```python
from build123d import *

# Parameters (mm, degrees)
F0_W     = 15
F0_H     = 15
F1_DEPTH = 15
F2_SIZE  = 13
F3_R     = 5.25
F3_R_2   = 2.25
F4_DEPTH = 5
F5_DEPTH = 3


with BuildPart() as f1:
    # F0 (on Top) → F1 (new body)
    with BuildSketch(Plane.XY):
        with Locations((7.5, -7.5)):
            Rectangle(F0_W, F0_H)
    extrude(amount=F1_DEPTH)

    # F2
    f2_edges = [f1.edges().sort_by_distance(p)[0] for p in [
        (15, -7.5, 15),
    ]]
    chamfer(f2_edges, length=F2_SIZE)

    # F3 (on face) → F4 (cut)
    with BuildSketch(Plane(origin=(8.5, 0, 8.5), x_dir=(0, 1, 0), z_dir=(0.7071067812, 0, 0.7071067812))):
        with Locations((-7.5, 0)):
            Circle(F3_R)
        with Locations((-7.5, 0)):
            Circle(F3_R_2, mode=Mode.SUBTRACT)
    extrude(amount=-F4_DEPTH, mode=Mode.SUBTRACT)

    # F5 (cut): a face of the model
    f5_faces = [f1.faces().sort_by_distance(p)[0] for p in [
        (8.5, -7.5, 8.5),
    ]]
    extrude(f5_faces, amount=-F5_DEPTH, mode=Mode.SUBTRACT)


solid = f1.part
```
Work out the finished part from the listing and answer in its coordinate system (mm). A direction names the side the tool comes from. Give positions to 0.01 mm unless a question says otherwise; leave off trailing zeros. Write each loop counter-clockwise with the first axis right and the second up, starting at its lowest first coordinate (ties: lowest second). Pieces come first, ordered by that corner, then holes. Notation, with made-up numbers: (1, -13.75) - (20, -13.75) arc R19 ccw to (20, -7.75) - close; hole circle Ø4 at (0.5, 82.25). An arc over 180 degrees is marked (long way). Use one line per item in the form item = value.
1. Consider L1, parallel to Z at x = 3, y = -3.25; L2, parallel to Z at x = 2.25, y = -5.25; L3, parallel to Y at x = 4, z = 8. Determine where each line is inside the solid, lowest interval first.
Filled in:
L1 = 0 to 6.93, 7.36 to 14
L2 = 0 to 7.68, 8.96 to 14.75
L3 = -15 to -11.92, -3.08 to 0
2. A cutting plane is placed at A-A (y = -8.25). Write down the section's boundary in (x, z).
Filled in:
outline = (0, 0) - (15, 0) - (15, 2) - (12.17, 4.83) - (8.64, 1.29) - (6.46, 3.46) - (7.88, 4.88) - (4.88, 7.88) - (3.46, 6.46) - (1.29, 8.64) - (4.83, 12.17) - (2, 15) - (0, 15) - close
3. A cutting plane is placed at B-B (x = 13). Write down the section's boundary in (y, z).
Filled in:
outline = (-15, 0) - (0, 0) - (0, 4) - (-15, 4) - close
4. For faces 5 (the face through (6.36, -7.53, 6.4)), 6 (the face through (1, -7, 15)), determine the directions among +Z, -Z, +X, -X, +Y, -Y from which every point of the face is accessible in a straight line to the end or side of a thin tool.
Filled in:
face_5 = +Z, +X
face_6 = +Z, +X, -X, +Y, -Y
5. A cutting plane is placed at C-C (z = 12.5). Write down the section's boundary in (x, y), and give its area (3 significant figures).
Filled in:
outline = (0, -15) - (4.5, -15) - (4.5, 0) - (0, 0) - close
area = 67.5 mm^2
6. A cutting plane is placed at D-D (y = -2.5). Write down the section's boundary in (x, z).
Filled in:
outline = (0, 0) - (15, 0) - (15, 2) - (9.63, 7.37) - (6.1, 3.83) - (3.83, 6.1) - (7.37, 9.63) - (2, 15) - (0, 15) - close
7. Each of these flat-tipped pins is pushed along its axis until it touches: pin 1 Ø5 at (y, z) = (-8, 5) entering from +X; pin 2 Ø6 at (x, y) = (10, -9) entering from +Z. Where does it stop, or does it pass through?
Filled in:
pin_1 = 14.5
pin_2 = 6.55
8. Determine the mould class of faces 1 (the face through (6.56, -6.41, 3.37)), 2 (the face through (6, 0, 6)), 3 (the face through (15, -8, 1)), 4 (the face through (6, -15, 6)) for opening direction Y: released by +Y, released by -Y, zero draft, split by the parting line, or undercut.
Filled in:
face_1 = undercut
face_2 = released by +Y
face_3 = zero draft
face_4 = released by -Y
